Check sheet for the drawn part. Datum: minimum x, y, z corner. Units: mm. Give positions to 0.01 mm unless a question says otherwise; leave off trailing zeros. Loops run counter-clockwise (first coordinate to the right, second up) from the corner with the lowest first, then second, coordinate; pieces in that order, holes last. Notation, with made-up numbers: M -15,62.5 L 25,62.5 A22 cw 25,80.5 Z; hole C 57.25,-13.75 d5. An arc over 180 degrees is marked long. Write each question's results on one line, items separated by ' | '. Start each with the question number.
1. Go/stop test with a flat-tipped pin: pin 1 (1.5 mm diameter, centred on y = 43, z = 3.5, fed in from -X). Record where the tip stops, or that it passes through.
2. Sectioned sample at D-D on y = 17. Record the cut outline in (x, z).
3. Material ranges on line 1 along X through (y, z) = (38.5, 0.55); line 2 along X through (y, z) = (25, 1.75); line 3 along X through (y, z) = (56.5, 4.4), recorded low to high.
4. Sectioned sample at A-A on x = 70.5. Record the cut outline in (y, z).
5. Sectioned sample at C-C on y = 54. Record the cut outline in (x, z) (1 decimal).
6. Sectioned sample at B-B on z = 0.9. Record the cut outline in (x, y), and give its area (3 significant figures).
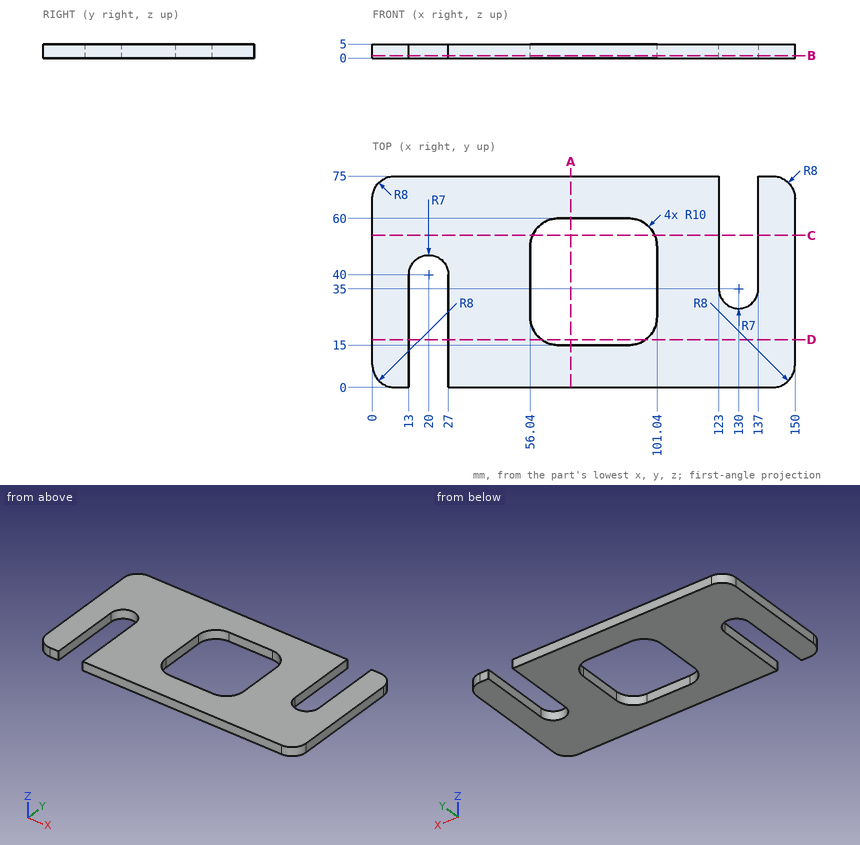
Output values:
1) pin 1: x = 0
2) outline: M 0,0 L 13,0 L 13,5 L 0,5 Z; M 27,0 L 60.04,0 L 60.04,5 L 27,5 Z; M 97.04,0 L 150,0 L 150,5 L 97.04,5 Z
3) line 1: 0 to 13, 27 to 56.04, 101.04 to 123, 137 to 150 | line 2: 0 to 13, 27 to 56.04, 101.04 to 150 | line 3: 0 to 58.44, 98.64 to 123, 137 to 150
4) outline: M 0,0 L 15,0 L 15,5 L 0,5 Z; M 60,0 L 75,0 L 75,5 L 60,5 Z
5) outline: M 0,0 L 56.9,0 L 56.9,5 L 0,5 Z; M 100.2,0 L 123,0 L 123,5 L 100.2,5 Z; M 137,0 L 150,0 L 150,5 L 137,5 Z
6) outline: M 0,8 A8 ccw 8,0 L 13,0 L 13,40 A7 cw 27,40 L 27,0 L 142,0 A8 ccw 150,8 L 150,67 A8 ccw 142,75 L 137,75 L 137,35 A7 cw 123,35 L 123,75 L 8,75 A8 ccw 0,67 Z; hole M 56.04,25 A10 ccw 66.04,15 L 91.04,15 A10 ccw 101.04,25 L 101.04,50 A10 ccw 91.04,60 L 66.04,60 A10 ccw 56.04,50 Z | area: 7,980 mm2
